Work out the finished part from the listing and answer in its coordinate system (mm). Coordinates: 2 decimals unless noted, no trailing zeros. Write each loop counter-clockwise with the first axis right and the second up, starting at its lowest first coordinate (ties: lowest second). Pieces come first, ordered by that corner, then holes. Notation, with made-up numbers: (24, -15) - (36, -15) arc R21 ccw to (36, 14) - close; hole circle Ø10 at (12.25, -20). An arc over 180 degrees is marked (long way). Use one line per item in the form item = value. Start each with the question number.
Item 1: Determine the mould class of faces 1 (the cylindrical face through (0, 0, 5)), 2 (the flat face through (8.5, -0.1, 5.5)), 3 (the cylindrical face through (-7.64, -9.6, 4.92)) for opening direction Y: released by +Y, released by -Y, zero draft, split by the parting line, or undercut.
Item 2: A cutting plane is placed at D-D (y = 6.75). Write down the section's boundary in (x, z).
Item 3: A cutting plane is placed at A-A (z = 6.6). Write down the section's boundary in (x, y) (3 decimals), then the cut area to 3 significant figures.
Item 4: A cutting plane is placed at B-B (x = 5). Write down the section's boundary in (y, z).
Item 5: Consider probe 1 along Y at (x, z) = (-5.5, 6.35) (3 decimals); probe 2 along Y at (x, z) = (5.5, 3.6) (3 decimals); probe 3 along X at (y, z) = (6.75, 5.3). Determine where each line is inside the solid, lowest interval first.
Item 6: A cutting plane is placed at C-C (z = 2.9). Write down the section's boundary in (x, y) (3 decimals).
from build123d import *

# Parameters (mm, degrees)
EXTRUDE_START       = 2
SKETCH_1_W          = 17
SKETCH_1_H          = 21
SKETCH_1_R          = 1.525
EXTRUDE_1_DEPTH     = 5.75
SKETCH_2_R          = 5
CUT_EXTRUDE_2_DEPTH = 22.43157717
FILLET_1_R          = 3


with BuildPart() as part:
    # 草图1 → 凸台-拉伸1 (new body)
    with BuildSketch(Plane.XY.offset(EXTRUDE_START)):
        Rectangle(SKETCH_1_W, SKETCH_1_H)
        with Locations((-5.5, 7.5)):
            Circle(SKETCH_1_R, mode=Mode.SUBTRACT)
        with Locations((5.5, 7.5)):
            Circle(SKETCH_1_R, mode=Mode.SUBTRACT)
        with Locations((5.5, -7.5)):
            Circle(SKETCH_1_R, mode=Mode.SUBTRACT)
        with Locations((-5.5, -7.5)):
            Circle(SKETCH_1_R, mode=Mode.SUBTRACT)
    extrude(amount=EXTRUDE_1_DEPTH)

    # 草图2 → 切除-拉伸2 (cut, through all)
    with BuildSketch(Plane(origin=(8.5, 0, 0), x_dir=(0, 0, -1), z_dir=(1, 0, 0))):
        Circle(SKETCH_2_R)
    extrude(amount=-CUT_EXTRUDE_2_DEPTH, mode=Mode.SUBTRACT)

    # 圆角1
    fillet_1_edges = [part.edges().sort_by_distance(p)[0] for p in [
        (-8.5, 10.5, 4.875),
        (8.5, 10.5, 4.875),
        (8.5, -10.5, 4.875),
        (-8.5, -10.5, 4.875),
    ]]
    fillet(fillet_1_edges, radius=FILLET_1_R)


solid = part.part
Answer:
q1.face_1 = undercut
q1.face_2 = zero draft
q1.face_3 = released by -Y
q2.outline = (-8.5, 2) - (-6.83, 2) - (-6.83, 7.75) - (-8.5, 7.75) - close; (-4.17, 2) - (4.17, 2) - (4.17, 7.75) - (-4.17, 7.75) - close; (6.83, 2) - (8.5, 2) - (8.5, 7.75) - (6.83, 7.75) - close
q3.outline = (-8.5, -7.5) arc R3 ccw to (-5.5, -10.5) - (5.5, -10.5) arc R3 ccw to (8.5, -7.5) - (8.5, 7.5) arc R3 ccw to (5.5, 10.5) - (-5.5, 10.5) arc R3 ccw to (-8.5, 7.5) - close; hole circle Ø3.05 at (-5.5, -7.5); hole circle Ø3.05 at (-5.5, 7.5); hole circle Ø3.05 at (5.5, -7.5); hole circle Ø3.05 at (5.5, 7.5)
q3.area = 320 mm²
q4.outline = (-10.5, 2) - (-8.94, 2) - (-8.94, 7.75) - (-10.5, 7.75) - close; (-6.06, 2) - (-4.58, 2) arc R5 cw to (4.58, 2) - (6.06, 2) - (6.06, 7.75) - (-6.06, 7.75) - close; (8.94, 2) - (10.5, 2) - (10.5, 7.75) - (8.94, 7.75) - close
q5.probe_1 = -10.5 to -9.025, -5.975 to 5.975, 9.025 to 10.5
q5.probe_2 = -10.5 to -9.025, -5.975 to -3.47, 3.47 to 5.975, 9.025 to 10.5
q5.probe_3 = -8.5 to -6.83, -4.17 to 4.17, 6.83 to 8.5
q6.outline = (-8.5, -7.5) arc R3 ccw to (-5.5, -10.5) - (5.5, -10.5) arc R3 ccw to (8.5, -7.5) - (8.5, -4.073) - (-8.5, -4.073) - close; (-8.5, 4.073) - (8.5, 4.073) - (8.5, 7.5) arc R3 ccw to (5.5, 10.5) - (-5.5, 10.5) arc R3 ccw to (-8.5, 7.5) - close; hole circle Ø3.05 at (-5.5, -7.5); hole circle Ø3.05 at (-5.5, 7.5); hole circle Ø3.05 at (5.5, -7.5); hole circle Ø3.05 at (5.5, 7.5)
